Design review of the part built by this model. Coordinates are the model's own, in mm. Face numbers are marked on the shaded views. Give positions to 0.01 mm unless a question says otherwise; leave off trailing zeros. Write each loop counter-clockwise with the first axis right and the second up, starting at its lowest first coordinate (ties: lowest second). Pieces come first, ordered by that corner, then holes. Notation, with made-up numbers: (41.25, 41.25) -> (86.25, 41.25) arc R4 ccw to (86.25, 46.25) -> close; hole circle Ø9 at (75.5, 75). An arc over 180 degrees is marked (long way). Return JSON: item names as keys, results as strings. Group by question number.
from build123d import *

# Parameters (mm, degrees)
SKETCH2_R           = 50
SKETCH2_R_2         = 12.5
BOSS_EXTRUDE1_DEPTH = 15
SKETCH6_R           = 5
CUT_EXTRUDE2_DEPTH  = 77.811457479
CIRPATTERN2_COUNT   = 6


with BuildPart() as part:
    # Sketch2 → Boss-Extrude1 (new, symmetric)
    with BuildSketch(Plane.XY):
        Circle(SKETCH2_R)
        Circle(SKETCH2_R_2, mode=Mode.SUBTRACT)
    extrude(amount=BOSS_EXTRUDE1_DEPTH, both=True)

    # Sketch6 → Cut-Extrude2 (cut, through all)
    with BuildSketch(Plane.XY.offset(15)):
        with Locations((0, 30)):
            Circle(SKETCH6_R)
    cut_extrude2 = extrude(amount=-CUT_EXTRUDE2_DEPTH, mode=Mode.SUBTRACT)

    # CirPattern2: Cut-Extrude2 ×6 about axis
    cirpattern2_axis = Axis((0, 0, 0), (0, 0, 1))
    for i in range(1, CIRPATTERN2_COUNT):
        add(cut_extrude2.rotate(cirpattern2_axis, i * 360 / CIRPATTERN2_COUNT), mode=Mode.SUBTRACT)


solid = part.part
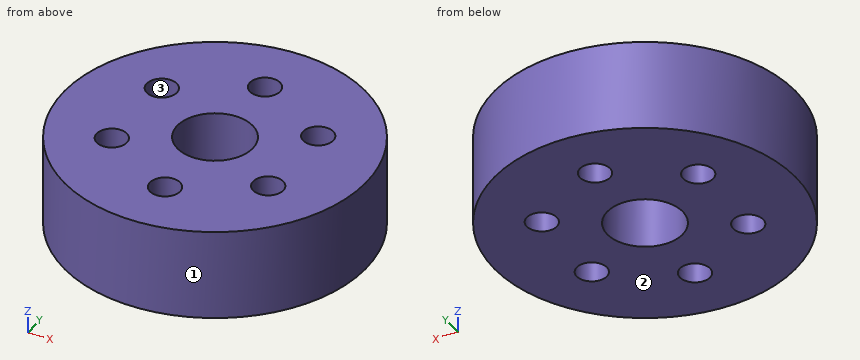
Q1. Mouldability with a two-part tool opening along X and no side actions: class the marked faces 1, 2 and 3 as +X half, -X half, draft (parallel to the pull), parting line (faces both ways), or undercut.
Q2. Take a section at B-B, the plane y = -30. Give the boundary of the cut face in (x, z), plus the area to 3 significant figures.
Q3. Insertion check: pin 1 (11.5 mm diameter, centred on x = 25.98, y = 15, fed in from +Z); pin 2 (8 mm diameter, centred on y = 9.5, z = -2.5, fed in from +X); pin 3 (1 mm diameter, centred on y = -35, z = 3, fed in from -X); pin 4 (8 mm diameter, centred on x = -25.98, y = 15, fed in from -Z). Each pin has a flat end and moves straight along its axis. Give the tip position at first contact, or say it passes through.
Q4. Take a section at D-D, the plane z = -9.5. Give the boundary of the cut face in (x, y), plus the area to 3 significant figures.
Q5. Take a section at A-A, the plane x = 0. Give the boundary of the cut face in (y, z), plus the area to 3 significant figures.
Q6. Take a section at C-C, the plane y = -15.5. Give the boundary of the cut face in (x, z), plus the area to 3 significant figures.
Q7. For L1, parallel to Y at x = 0, z = -3.5; L2, parallel to Y at x = -2, z = 8.75; L3, parallel to X at y = -11, z = 13.25 (3 decimals), list the stretches that pass through material, from the lowest coordinate up. Write a range as from..to.
Final values:
{
 "1": {"face 1": "parting line", "face 2": "draft", "face 3": "undercut"},
 "2": {"outline": "(-40, -15) -> (-5, -15) -> (-5, 15) -> (-40, 15) -> close; (5, -15) -> (40, -15) -> (40, 15) -> (5, 15) -> close", "area": "2,100 mm²"},
 "3": {"pin 1": "stops at z = 15", "pin 2": "stops at x = 49.7", "pin 3": "stops at x = -36.19", "pin 4": "passes through"},
 "4": {"outline": "circle Ø100 at (0, 0); hole circle Ø10 at (-25.98, -15); hole circle Ø10 at (-25.98, 15); hole circle Ø25 at (0, 0); hole circle Ø10 at (0, -30); hole circle Ø10 at (0, 30); hole circle Ø10 at (25.98, -15); hole circle Ø10 at (25.98, 15)", "area": "6,890 mm²"},
 "5": {"outline": "(-50, -15) -> (-35, -15) -> (-35, 15) -> (-50, 15) -> close; (-25, -15) -> (-12.5, -15) -> (-12.5, 15) -> (-25, 15) -> close; (12.5, -15) -> (25, -15) -> (25, 15) -> (12.5, 15) -> close; (35, -15) -> (50, -15) -> (50, 15) -> (35, 15) -> close", "area": "1,650 mm²"},
 "6": {"outline": "(-47.54, -15) -> (-30.96, -15) -> (-30.96, 15) -> (-47.54, 15) -> close; (-21.01, -15) -> (21.01, -15) -> (21.01, 15) -> (-21.01, 15) -> close; (30.96, -15) -> (47.54, -15) -> (47.54, 15) -> (30.96, 15) -> close", "area": "2,260 mm²"},
 "7": {"L1": "y = -50..-35, -25..-12.5, 12.5..25, 35..50", "L2": "y = -49.96..-34.58, -25.42..-12.34, 12.34..25.42, 34.58..49.96", "L3": "x = -48.775..-28.981, -22.981..-5.937, 5.937..22.981, 28.981..48.775"}
}
